```python
from build123d import *

# Parameters (mm, degrees)
SKETCH1_R           = 12
BOSS_EXTRUDE1_DEPTH = 35
DOME1_FACE_RADIUS   = 12
DOME1_HEIGHT        = 12


# Read off the part's stored shape, not the designer's step: Shell1
with BuildPart() as part:
    # Sketch1 → Boss-Extrude1 (new body)
    with BuildSketch(Plane.XY):
        Circle(SKETCH1_R)
    extrude(amount=BOSS_EXTRUDE1_DEPTH)

    # Dome1: a dome of height H over a round flat face of radius A is a cap of a sphere of radius (A * A + H * H) / (2 * H)
    dome1_r = (DOME1_FACE_RADIUS * DOME1_FACE_RADIUS + DOME1_HEIGHT * DOME1_HEIGHT) / (2 * DOME1_HEIGHT)
    dome1_base = Plane((0, 0, 35), z_dir=(0, 0, 1))
    with Locations(dome1_base.offset(DOME1_HEIGHT - dome1_r)):
        dome1_ball = Sphere(dome1_r, mode=Mode.PRIVATE)
    add(split(dome1_ball, bisect_by=dome1_base, keep=Keep.TOP, mode=Mode.PRIVATE))

    # Shell1 outline → Shell1 (revolve, cut)
    with BuildSketch(Plane.XZ):
        with BuildLine():
            Line((10.5, 1.5), (10.5, 34.999999989))
            ThreePointArc((10.5, 34.999999989), (7.424621206, 42.424621199), (0, 45.5))
            Line((0, 45.5), (0, 1.5))
            Line((0, 1.5), (10.5, 1.5))
        make_face()
    revolve(axis=Axis((0, 0, 0), (0, 0, 1)), mode=Mode.SUBTRACT)


solid = part.part
```
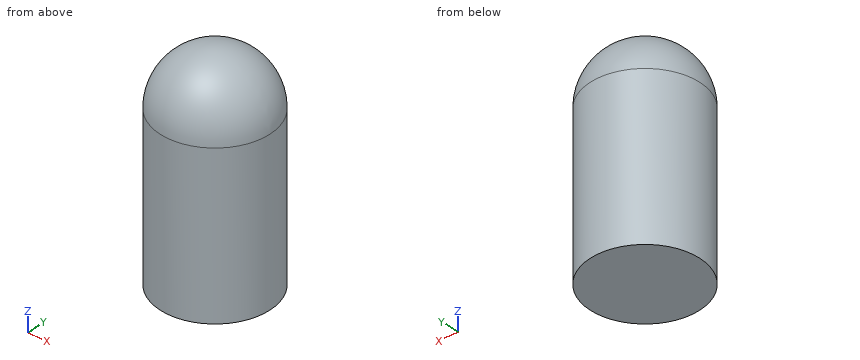
Can you work these out from the model? Positions are in its coordinate system, mm. Round coordinates to 2 decimals unless told otherwise and drop trailing zeros. Loops run counter-clockwise (first coordinate to the right, second up) from the corner with the lowest first, then second, coordinate; pieces in that order, holes last. Notation, with made-up numbers: (55, 65) -> (67, 65) arc R22 cw to (67, 96) -> close; hole circle Ø9 at (21, 71.25). An arc over 180 degrees is marked (long way). Answer in a Markdown table with one row per item.
Item 1: Suppose I cut it at C-C, the plane z = 27.5. List the corners of the cut face in (x, y) for me, plus the area to 3 significant figures.
Answer block:
| item | result |
|---|---|
| outline | circle Ø24 at (0, 0); hole circle Ø21 at (0, 0) |
| area | 106 mm² |
Item 2: Will these pins go through, and if not, where does the flat tip stop? P1, Ø10, axis at y = 5.5, z = 5.5, coming from the +X side; P2, Ø5, axis at x = -3, z = 18, coming from the -Y side; P3, Ø6, axis at y = 5.5, z = 15.5, coming from the -X side.
Answer block:
| item | result |
|---|---|
| P1 | x = 11.99 |
| P2 | y = -11.99 |
| P3 | x = -11.74 |
Item 3: Suppose I cut it at D-D, the plane y = -9. List the corners of the cut face in (x, z) for me, plus the area to 3 significant figures.
Answer block:
| item | result |
|---|---|
| outline | (-7.94, 0) -> (7.94, 0) -> (7.94, 35) arc R7.94 ccw to (-7.94, 35) -> close; hole (-5.41, 1.5) -> (5.41, 1.5) -> (5.41, 35) arc R5.41 ccw to (-5.41, 35) -> close |
| area | 246 mm² |
Item 4: If I drill on probe 1 along Y at (x, z) = (0, 26.5); probe 2 along Z at (x, y) = (-1.5, -3); probe 3 along Z at (x, y) = (2.5, -3), over which ranges is the centre line in solid material (lowest first)?
Answer block:
| item | result |
|---|---|
| probe 1 | -12 to -10.5, 10.5 to 12 |
| probe 2 | 0 to 1.5, 44.95 to 46.52 |
| probe 3 | 0 to 1.5, 44.75 to 46.35 |
Item 5: Suppose I cut it at A-A, the plane y = 0. List the corners of the cut face in (x, z) for me, plus the area to 3 significant figures.
Answer block:
| item | result |
|---|---|
| outline | (-12, 0) -> (12, 0) -> (12, 35) arc R12 ccw to (-12, 35) -> close; hole (-10.5, 1.5) -> (10.5, 1.5) -> (10.5, 35) arc R10.5 ccw to (-10.5, 35) -> close |
| area | 190 mm² |
